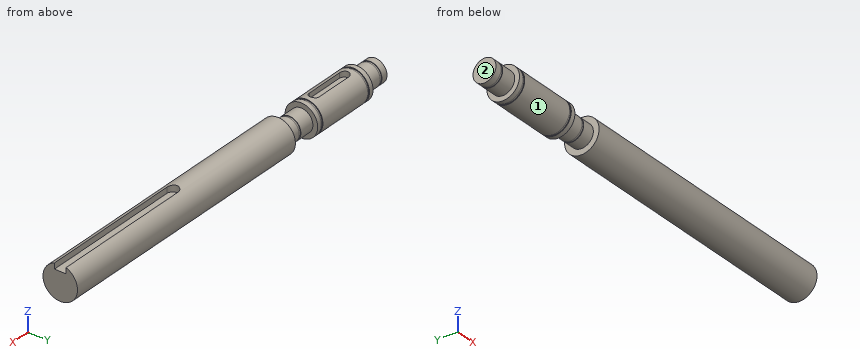
```python
from build123d import *

# Parameters (mm, degrees)
F4_DEPTH = 3
F7_DEPTH = 3.5


with BuildPart() as f1:
    # F0 (on Front) → F1 (revolve)
    with BuildSketch(Plane.XZ):
        Polygon((2.250003, 6), (2.250003, 0), (64.250003, 0), (81.750003, 0), (192.750003, 0), (212.750003, 0), (212.750003, 6), (212.750003, 9), (192.750003, 9), (67.250003, 9), (67.250003, 6), (62.250003, 6), (60.850003, 6), (60.850003, 5.75), (59.750003, 5.75), (59.750003, 6), (51.750003, 6), (51.750003, 8.5), (49.350003, 8.5), (49.350003, 8.1), (48.250003, 8.1), (48.250003, 8.5), (18.250003, 8.5), (18.250003, 8.1), (17.150003, 8.1), (17.150003, 8.5), (14.750003, 8.5), (14.750003, 6), (6.750003, 6), (6.750003, 5.75), (5.650003, 5.75), (5.650003, 6), align=None)
    revolve(axis=Axis((33.250003, 0, 0), (1, 0, 0)))

    # F3 (on offset) → F4 (cut)
    with BuildSketch(Plane.XY.offset(8.5)):
        with BuildLine():
            Line((43.250003, 2.5), (23.250003, 2.5))
            ThreePointArc((23.250003, 2.5), (20.750003, 0), (23.250003, -2.5))
            Line((23.250003, -2.5), (43.250003, -2.5))
            ThreePointArc((43.250003, -2.5), (45.750003, 0), (43.250003, 2.5))
        make_face()
    extrude(amount=-F4_DEPTH, mode=Mode.SUBTRACT)

    # F6 (on offset) → F7 (cut)
    with BuildSketch(Plane.XY.offset(9)):
        with BuildLine():
            Line((212.750003, 3), (137.750003, 3))
            ThreePointArc((137.750003, 3), (134.750003, 0), (137.750003, -3))
            Line((137.750003, -3), (212.750003, -3))
            Line((212.750003, -3), (212.750003, 3))
        make_face()
    extrude(amount=-F7_DEPTH, mode=Mode.SUBTRACT)


solid = f1.part
```
Read the model definition and answer for the solid it produces. Units are mm, in the model's axes. Face numbers are marked on the shaded views. A direction names the side the tool comes from. Coordinates: 2 decimals unless noted, no trailing zeros. Write each loop counter-clockwise with the first axis right and the second up, starting at its lowest first coordinate (ties: lowest second). Pieces come first, ordered by that corner, then holes. Notation, with made-up numbers: (53.25, 18.25) - (102.25, 18.25) arc R21 ccw to (102.25, 44.25) - close; hole circle Ø9 at (43.5, 52.25). An arc over 180 degrees is marked (long way). Answer as a JSON object with one key per item and string values. Group by question number.
1. Each of these flat-tipped pins is pushed along its axis until it touches: P1, Ø5, axis at x = 23.5, y = 4.5, coming from the +Z side; P2, Ø0.9, axis at x = 158, z = 7, coming from the -Y side; P3, Ø2.5, axis at x = 37.5, y = 0, coming from the +Z side. Where does it stop, or does it pass through?
2. A cutting plane is placed at A-A (x = 129). Determine the outline of the cut face in (y, z), plus the area to 3 significant figures.
3. Which of the six approach directions +Z, -Z, +X, -X, +Y, -Y give full straight-line access (tool end or side, diameter ignored) to the marked faces 1 and 2?
4. A cutting plane is placed at B-B (x = 56.5). Determine the outline of the cut face in (y, z), plus the area to 3 significant figures.
5. Consider L1, parallel to X at y = 6.5, z = 1.25; L2, parallel to Z at x = 38, y = -0.25; L3, parallel to X at y = -6.5, z = 6. Determine where each line is inside the solid, lowest interval first. Write a range as [from, to].
Worked out:
{
 "1": {"P1": "stops at z = 8.18", "P2": "stops at y = -6.17", "P3": "stops at z = 5.5"},
 "2": {"outline": "circle Ø18 at (0, 0)", "area": "254 mm²"},
 "3": {"face 1": "-X", "face 2": "+Z, -Z, -X, +Y, -Y"},
 "4": {"outline": "circle Ø12 at (0, 0)", "area": "113 mm²"},
 "5": {"L1": "x = [14.75, 51.75], [67.25, 212.75]", "L2": "z = [-8.5, 5.5]", "L3": "x = [67.25, 212.75]"}
}
